from build123d import *

# Parameters (mm, degrees)
CROQUIS1_R              = 2.65
CROQUIS1_R_2            = 3.72
SALIENTE_EXTRUIR2_DEPTH = 8
CORTAR_EXTRUIR1_START   = 8
CROQUIS1_4_R            = 5.05
CROQUIS1_4_R_2          = 6
CORTAR_EXTRUIR1_DEPTH   = 2.8


with BuildPart() as part:
    # Croquis1 → Saliente-Extruir2 (new body)
    with BuildSketch(Plane(origin=(0, 0, 0), x_dir=(1, 0, 0), z_dir=(0, 1, 0))):
        with BuildLine():
            Line((-20, -25), (20, -25))
            ThreePointArc((20, -25), (23.535533906, -23.535533906), (25, -20))
            Line((25, -20), (25, 20))
            ThreePointArc((25, 20), (23.535533906, 23.535533906), (20, 25))
            Line((20, 25), (-20, 25))
            ThreePointArc((-20, 25), (-23.535533906, 23.535533906), (-25, 20))
            Line((-25, 20), (-25, -20))
            ThreePointArc((-25, -20), (-23.535533906, -23.535533906), (-20, -25))
        make_face()
        with Locations((-12.5, -15)):
            Circle(CROQUIS1_R, mode=Mode.SUBTRACT)
        with Locations((-12.5, 15)):
            Circle(CROQUIS1_R_2, mode=Mode.SUBTRACT)
        with Locations((0, -17)):
            Circle(CROQUIS1_R, mode=Mode.SUBTRACT)
        with Locations((-17, 0)):
            Circle(CROQUIS1_R, mode=Mode.SUBTRACT)
        with Locations((0, 17)):
            Circle(CROQUIS1_R, mode=Mode.SUBTRACT)
        with Locations((17, 0)):
            Circle(CROQUIS1_R, mode=Mode.SUBTRACT)
        with Locations((12.5, -15)):
            Circle(CROQUIS1_R, mode=Mode.SUBTRACT)
        with Locations((12.5, 15)):
            Circle(CROQUIS1_R_2, mode=Mode.SUBTRACT)
        with BuildLine():
            Line((-7.060224725, -6.03567091), (7.060224725, -6.03567091))
            ThreePointArc((7.060224725, -6.03567091), (9.181545068, -5.156991253), (10.060224725, -3.03567091))
            Line((10.060224725, -3.03567091), (10.060224725, 3.03567091))
            ThreePointArc((10.060224725, 3.03567091), (9.181545068, 5.156991253), (7.060224725, 6.03567091))
            Line((7.060224725, 6.03567091), (-7.060224725, 6.03567091))
            ThreePointArc((-7.060224725, 6.03567091), (-9.181545068, 5.156991253), (-10.060224725, 3.03567091))
            Line((-10.060224725, 3.03567091), (-10.060224725, -3.03567091))
            ThreePointArc((-10.060224725, -3.03567091), (-9.181545068, -5.156991253), (-7.060224725, -6.03567091))
        make_face(mode=Mode.SUBTRACT)
    extrude(amount=SALIENTE_EXTRUIR2_DEPTH)

    # Croquis1<4> → Cortar-Extruir1 (cut)
    with BuildSketch(Plane(origin=(0, 0, 0), x_dir=(1, 0, 0), z_dir=(0, 1, 0)).offset(CORTAR_EXTRUIR1_START)):
        with Locations((-12.5, -15)):
            Circle(CROQUIS1_4_R)
        with Locations((-12.5, 15)):
            Circle(CROQUIS1_4_R_2)
        with Locations((12.5, -15)):
            Circle(CROQUIS1_4_R)
        with Locations((12.5, 15)):
            Circle(CROQUIS1_4_R_2)
    extrude(amount=-CORTAR_EXTRUIR1_DEPTH, mode=Mode.SUBTRACT)


solid = part.part
Geometry check sheet. Reference: the model listing, model coordinates, mm. A direction names the side the tool comes from. Round coordinates to 2 decimals unless told otherwise and drop trailing zeros. Loops run counter-clockwise (first coordinate to the right, second up) from the corner with the lowest first, then second, coordinate; pieces in that order, holes last. Notation, with made-up numbers: (-17, 11.25) - (-1, 11.25) arc R28 cw to (-1, 37.25) - close; hole circle Ø6 at (13.5, -19). An arc over 180 degrees is marked (long way). One line per question, with ' | ' between items. Start each with the question number.
1. Draft check along Z on faces 4 (the face through (15, 5.2, 17)), 5 (the face through (23, 4, 24)), 6 (the face through (0, 4, -25)). Enter one of: released by +Z, released by -Z, zero draft, split by the parting line, or undercut.
2. Depth check by flat-ended pin: pin 1 (5 mm diameter, centred on x = -12, z = 17, fed in from +Y); pin 2 (3 mm diameter, centred on x = -12.5, z = 15, fed in from +Y) (3 decimals). Enter the tip coordinate at first touch or a pass-through.
3. Cross-section at B-B on y = 6. State how many separate pieces and enclosed holes the cut face has, then the cut area to 3 significant figures.
4. Cross-section at A-A on x = 0. Record the cut outline in (y, z).
5. Cross-section at C-C on z = 0. Record the cut outline in (x, y), then the cut area to 3 significant figures.
6. Scan lines: line 1 (Z direction, x = -12.5, y = 3.85); line 2 (X direction, y = 4.25, z = 0); line 3 (Z direction, x = 0, y = 1). Record each from-to range of solid material in increasing order. Write a range as [from, to].
7. Tool access check on faces 1 (the face through (-24, 4, 23)), 2 (the face through (-9.16, 3.94, -5.18)), 3 (the face through (17.317, 6.62, 13.483)). Record the directions out of +Z, -Z, +X, -X, +Y, -Y that give a thin tool (end or side, any length) a straight path to the whole face; none if there is none.
8. Cross-section at D-D on x = 12.5. Record the cut outline in (y, z), then the cut area to 3 significant figures.
Taken from the geometry:
1) face 4: undercut | face 5: released by +Z | face 6: released by -Z
2) pin 1: y = 5.2 | pin 2: through
3) separate pieces: 1 | enclosed holes: 9 | area: 1,770 mm²
4) outline: (0, -25) - (8, -25) - (8, -19.65) - (0, -19.65) - close; (0, -14.35) - (8, -14.35) - (8, -6.04) - (0, -6.04) - close; (0, 6.04) - (8, 6.04) - (8, 14.35) - (0, 14.35) - close; (0, 19.65) - (8, 19.65) - (8, 25) - (0, 25) - close
5) outline: (-25, 0) - (-19.65, 0) - (-19.65, 8) - (-25, 8) - close; (-14.35, 0) - (-10.06, 0) - (-10.06, 8) - (-14.35, 8) - close; (10.06, 0) - (14.35, 0) - (14.35, 8) - (10.06, 8) - close; (19.65, 0) - (25, 0) - (25, 8) - (19.65, 8) - close | area: 154 mm²
6) line 1: [-25, -18.72], [-11.28, 12.35], [17.65, 25] | line 2: [-25, -19.65], [-14.35, -10.06], [10.06, 14.35], [19.65, 25] | line 3: [-25, -19.65], [-14.35, -6.04], [6.04, 14.35], [19.65, 25]
7) face 1: +Z, -X, +Y, -Y | face 2: +Y, -Y | face 3: +Y
8) outline: (0, -25) - (8, -25) - (8, -21) - (5.2, -21) - (5.2, -18.72) - (0, -18.72) - close; (0, -11.28) - (5.2, -11.28) - (5.2, -9) - (8, -9) - (8, 9.95) - (5.2, 9.95) - (5.2, 12.35) - (0, 12.35) - close; (0, 17.65) - (5.2, 17.65) - (5.2, 20.05) - (8, 20.05) - (8, 25) - (0, 25) - close | area: 272 mm²
